Check sheet for the modelled part. Datum: model origin and axes. Units: mm. A direction names the side the tool comes from. Round coordinates to 2 decimals unless told otherwise and drop trailing zeros. Loops run counter-clockwise (first coordinate to the right, second up) from the corner with the lowest first, then second, coordinate; pieces in that order, holes last. Notation, with made-up numbers: (61, -9) - (117, -9) arc R26 ccw to (117, 20) - close; hole circle Ø9 at (21.25, 59.25). An arc over 180 degrees is marked (long way). Put each result on its own line as item: value. Start each with the question number.
```python
from build123d import *

# Parameters (mm, degrees)
BOSS_EXTRUDE1_DEPTH = 25.4
FILLET1_R           = 1.27


with BuildPart() as part:
    # Sketch1 → Boss-Extrude1 (new body)
    with BuildSketch(Plane.XY):
        with BuildLine():
            Line((0, 0), (0, 35.56))
            Line((0, 35.56), (0, 57.15))
            Line((0, 57.15), (10.16, 57.15))
            Line((10.16, 57.15), (10.16, 38.1))
            ThreePointArc((10.16, 38.1), (10.903948776, 36.303948776), (12.7, 35.56))
            Line((12.7, 35.56), (33.02, 35.56))
            Line((33.02, 35.56), (33.02, 25.4))
            Line((33.02, 25.4), (12.192, 25.4))
            ThreePointArc((12.192, 25.4), (10.755159021, 24.804840979), (10.16, 23.368))
            Line((10.16, 23.368), (10.16, 0))
            Line((10.16, 0), (0, 0))
        make_face()
    extrude(amount=BOSS_EXTRUDE1_DEPTH)

    # Fillet1
    fillet1_edges = [part.edges().sort_by_distance(p)[0] for p in [
        (0, 0, 12.7),
        (0, 57.15, 12.7),
        (0, 28.575, 0),
        (5.08, 0, 0),
        (10.16, 47.625, 0),
        (10.903948776, 36.303948776, 0),
        (22.86, 35.56, 0),
        (5.08, 57.15, 0),
        (33.02, 35.56, 12.7),
        (33.02, 30.48, 0),
    ]]
    fillet(fillet1_edges, radius=FILLET1_R)


solid = part.part
```
Q1. Set-up check for faces 1 (the face through (9.798, 47.492, 0.382)), 2 (the face through (23, 25.4, 13)), 3 (the face through (10.16, 48, 13)): record each of +Z, -Z, +X, -X, +Y, -Y from which the full face is reachable in a straight line by a thin tool's end or side.
Q2. Cross-section at A-A on z = 7.75. Enter the section's corners in (x, y), and give its area (3 significant figures).
Q3. Cross-section at D-D on y = 52. Enter the section's corners in (x, z).
Q4. Cross-section at C-C on y = 9. Enter the section's corners in (x, z), and give its area (3 significant figures).
Q5. Cross-section at B-B on x = 23. Enter the section's corners in (y, z), and give its area (3 significant figures).
Q6. Material ranges on line 1 (Y direction, x = 19.5, z = 10.75); line 2 (X direction, y = 14, z = 9.25); line 3 (X direction, y = 35, z = 16.75), recorded low to high. Write a range as from..to.
Q7. Depth check by flat-ended pin: pin 1 Ø7 at (y, z) = (7.5, 8) entering from +X; pin 2 Ø10 at (x, z) = (17.5, 20.5) entering from -Y; pin 3 Ø9.5 at (x, z) = (20.5, 9) entering from +Y. Enter the tip coordinate at first touch or a pass-through.
Answer list:
1. face 1: -Z, +X, +Y
1. face 2: +Z, -Z, +X, -Y
1. face 3: +Z, -Z, +X, +Y
2. outline: (0, 1.27) arc R1.27 ccw to (1.27, 0) - (10.16, 0) - (10.16, 23.37) arc R2.03 cw to (12.19, 25.4) - (33.02, 25.4) - (33.02, 34.29) arc R1.27 ccw to (31.75, 35.56) - (12.7, 35.56) arc R2.54 cw to (10.16, 38.1) - (10.16, 57.15) - (1.27, 57.15) arc R1.27 ccw to (0, 55.88) - close
2. area: 814 mm2
3. outline: (0, 1.27) arc R1.27 ccw to (1.27, 0) - (8.89, 0) arc R1.27 ccw to (10.16, 1.27) - (10.16, 25.4) - (0, 25.4) - close
4. outline: (0, 1.27) arc R1.27 ccw to (1.27, 0) - (10.16, 0) - (10.16, 25.4) - (0, 25.4) - close
4. area: 258 mm2
5. outline: (25.4, 0) - (34.29, 0) arc R1.27 ccw to (35.56, 1.27) - (35.56, 25.4) - (25.4, 25.4) - close
5. area: 258 mm2
6. line 1: y = 25.4..35.56
6. line 2: x = 0..10.16
6. line 3: x = 0..32.8
7. pin 1: stops at x = 10.16
7. pin 2: stops at y = 25.4
7. pin 3: stops at y = 35.56
